Geometry check sheet. Reference: the model listing, model coordinates, mm. A direction names the side the tool comes from. Coordinates: 2 decimals unless noted, no trailing zeros. Write each loop counter-clockwise with the first axis right and the second up, starting at its lowest first coordinate (ties: lowest second). Pieces come first, ordered by that corner, then holes. Notation, with made-up numbers: M 70.5,74.5 L 121.5,74.5 A27 cw 121.5,103.5 Z; hole C -34.75,88.25 d6. An arc over 180 degrees is marked long. Write item = value, one per line. Start each with the question number.
Autodesk Inventor part; units mm, degrees
ref_plane "YZ Plane" through (0, 0, 0) normal (1, 0, 0) x (0, 1, 0)
ref_plane "XZ Plane" through (0, 0, 0) normal (0, 1, 0) x (-1, 0, 0)
ref_plane "XY Plane" through (0, 0, 0) normal (0, 0, 1) x (1, 0, 0)
sketch "Sketch1" plane through (0, 0, 0) normal (0, 1, 0) x (-1, 0, 0)
  arc A0 (52.6783, -85) -> (52.6783, 85) centre (0, 0) ccw
  circle A1 centre (130, 70) radius 3
  circle A2 centre (130, -70) radius 3
  line L0 (52.6783, 85) -> (135, 85)
  line L1 (52.6783, -85) -> (135, -85)
  line L2 (135, -85) -> (135, 85)
  circle A3 centre (72.25, 0) radius 25.25
  circle A4 centre (72.25, 0) radius 27.75
  arc A5 (47.7624, -85) -> (47.7624, 85) centre (0, 0) ccw
  line L3 (52.6783, 85) -> (47.7624, 85)
  line L4 (52.6783, -85) -> (47.7624, -85)
  point P0 (100, 0)
  point P1 (96.583, -13.3404)
  point P2 (96.583, 13.3404)
  dimension "d9" = 6
  dimension "d10" = 6
  dimension "d29" = 50.5
  dimension "d30" = 55.5
extrude "Extrusion1" add sketch "Sketch1" along normal blind 3 contours A0 L0 L2 L1 | A3
extrude "Extrusion3" add sketch "Sketch1" along normal blind 3 and the other way blind 20 contours A4 A5 | A5 A4
extrude "Extrusion4" add sketch "Sketch1" along normal blind 3 and the other way blind 6 contours L4 A5 A4 A0 | A4 A5 L3 A0
sketch "Sketch3" plane through (0, -6, 0) normal (0, -1, 0) x (1, 0, 0)
  arc A0 (-96.583, -13.3404) -> (-47.7624, -85) centre (0, 0) ccw
  line L0 (0, 0) -> (-135, 0)
  line L1 (-135, -85) -> (-135, 85)
  line L2 (-135, 0) -> (-135, 85)
  line L3 (-135, 85) -> (-47.7624, 85)
  line L4 (-135, 85) -> (-47.7624, 85)
  line L5 (-47.7624, -85) -> (-135, -85)
  line L6 (-135, 0) -> (-135, -85)
  line L7 (-135, -85) -> (-47.7624, -85)
  arc A1 (-47.7624, 85) -> (-47.7624, -85) centre (0, 0) ccw
  circle A2 centre (-130, -70) radius 3
  circle A3 centre (-130, -70) radius 3
  circle A4 centre (-130, 70) radius 3
  circle A5 centre (-130, 70) radius 3
  point P0 (-96.583, -13.3404)
  dimension "d40" = 135
extrude "Extrusion5" add sketch "Sketch3" along normal blind 5
sketch "Sketch6" plane through (-72.25, 0, 0) normal (0, -1, 0) x (1, 0, 0)
  circle A0 centre (0, 0) radius 25.25
  point P0 (72.25, 0)
extrude "Extrusion6" add sketch "Sketch6" along normal blind 2
sketch "Sketch7" plane through (0, 3, 0) normal (0, 1, 0) x (1, 0, 0)
  arc A0 (-96.583, -13.3404) -> (-96.583, 13.3404) centre (-72.25, 0) ccw
  line L0 (-72.25, 0) -> (-72.25, -12)
  line L1 (-72.25, -12) -> (-60.25, -12)
  line L2 (-60.25, -12) -> (-60.25, 12)
  line L3 (-60.25, 12) -> (-84.25, 12)
  line L4 (-84.25, 12) -> (-84.25, -12)
  point P0 (0, 0)
  dimension "d57" = 12
  dimension "d58" = 12
  dimension "d59" = 24
  dimension "d60" = 24
  dimension "d61" = 24
hole "Hole2" at (-60.25, 3, 12) at (-60.25, 3, -12) at (-84.25, 3, -12) at (-84.25, 3, 12) direction (0, -1, 0) diameter 3.5 end through all counterbore diameter 5.5 counterbore depth 3
fillet "Fillet1" radius 10 2 edges at (-96.583, -4, -13.3404) (-96.583, -4, 13.3404)
properties part number "ECHO SOUNDER HOLDER FINAL DESIGN (revised)"
Q1. Gauge pin test, flat ends, axial feed: pin 1 (2 mm diameter, centred on x = -96.5, y = -13.5, fed in from -Z); pin 2 (6.5 mm diameter, centred on x = -60.25, z = 12, fed in from -Y); pin 3 (4.5 mm diameter, centred on x = -60, z = -12, fed in from +Y). Record the tip position at first contact, or that the pin passes through.
Q2. Set-up check for faces 1 (the face through (-132.77, 1.48, 71.15)), 2 (the face through (-113, -6, 1)), 3 (the face through (-85.08, 1.48, -9.38)), 4 (the face through (-47.024, -10.874, 1.11)): record each of +Z, -Z, +X, -X, +Y, -Y from which the full face is reachable in a straight line by a thin tool's end or side.
Q3. Draft check along Z on faces 5 (the face through (-111, -11, 1)), 6 (the face through (-73, -2, 0)), 7 (the face through (-99.99, -3.04, 1.42)). Enter one of: pulls with the +Z half, pulls with the -Z half, needs draft (parallel to the pull), parting line crosses it, or undercut.
Q4. Scan lines: L1, parallel to Z at x = -130, y = -7.2; L2, parallel to X at y = -0.6, z = 12; L3, parallel to X at y = 0.85, z = 12. Record each from-to range of solid material in increasing order.
Q5. Cross-section at D-D on z = 49.5. Enter the section's corners in (x, y), and give its area (3 significant figures).
Q6. Cross-section at B-B on y = -18. Enter the section's corners in (x, z), and give its area (3 significant figures).
Q7. Cross-section at C-C on x = -72.25. Enter the section's corners in (y, z), and give its area (3 significant figures).
Q8. Cross-section at A-A on x = -123.5. Enter the section's corners in (y, z), and give its area (3 significant figures).
Values found:
q1.pin_1 = -15.15
q1.pin_2 = -2
q1.pin_3 = 0
q2.face_1 = +Y, -Y
q2.face_2 = -X
q2.face_3 = +Y
q2.face_4 = -Y
q3.face_5 = needs draft
q3.face_6 = undercut
q3.face_7 = parting line crosses it
q4.L1 = -85 to -73, -67 to 67, 73 to 85
q4.L2 = -99.28 to -86, -82.5 to -62, -58.5 to -47.23
q4.L3 = -135 to -87, -81.5 to -63, -57.5 to -47.23
q5.outline = M -135,-11 L -84,-11 L -84,3 L -135,3 L -135,0 L -86.89,0 L -86.89,-6 L -135,-6 Z
q5.area = 425 mm²
q6.outline = C -72.25,0 d55.5; hole C -72.25,0 d50.5
q6.area = 416 mm²
q7.outline = M -20,-27.75 L 3,-27.75 L 3,27.75 L -20,27.75 L -20,25.25 L -2,25.25 L -2,-25.25 L -20,-25.25 Z; M -11,-85 L -6,-85 L -6,-69.14 L 0,-69.14 L 0,-85 L 3,-85 L 3,-65.47 L -11,-65.47 Z; M -11,65.47 L 3,65.47 L 3,85 L 0,85 L 0,69.14 L -6,69.14 L -6,85 L -11,85 Z
q7.area = 724 mm²
q8.outline = M -11,-85 L -6,-85 L -6,85 L -11,85 Z; M 0,-85 L 3,-85 L 3,85 L 0,85 Z
q8.area = 1,360 mm²
